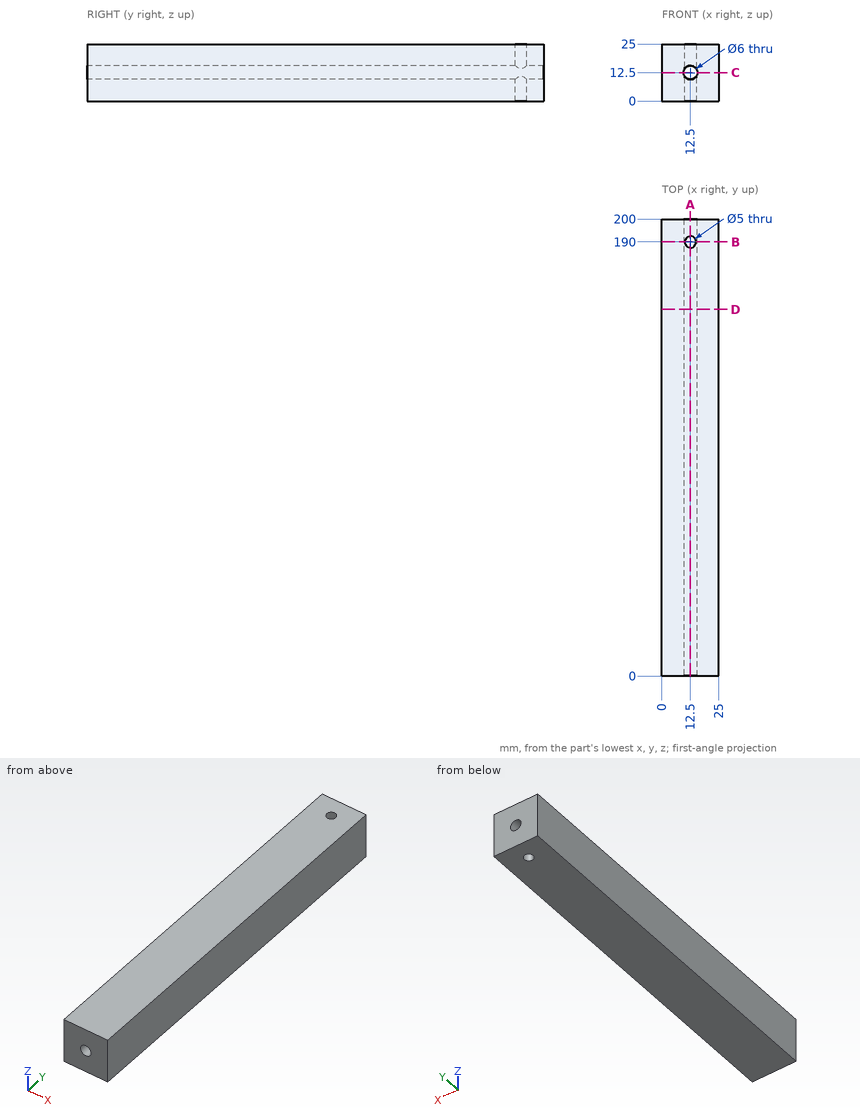
Part print with two shaded views. Sizes in mm from the minimum x, y, z corner. Coordinates: 2 decimals unless noted, no trailing zeros. Write each loop counter-clockwise with the first axis right and the second up, starting at its lowest first coordinate (ties: lowest second). Pieces come first, ordered by that corner, then holes. Notation, with made-up numbers: (15.25, 89.5) - (67.25, 89.5) arc R9 cw to (67.25, 100.5) - close; hole circle Ø2 at (42.5, 9). An arc over 180 degrees is marked (long way). Put each result on its own line as item: value.
1. Band-saw the part on B-B (y = 190). Write the cut outline in (x, z), then the cut area to 3 significant figures.
Final values:
outline: (0, 0) - (10, 0) - (10, 10.84) arc R3 cw to (10, 14.16) - (10, 25) - (0, 25) - close; (15, 0) - (25, 0) - (25, 25) - (15, 25) - (15, 14.16) arc R3 cw to (15, 10.84) - close
area: 498 mm²
2. Flat gauge pin, fed straight in: pin 1 Ø4.5 at (x, y) = (12.5, 190) entering from -Z. Where does the tip first touch, or does it go through?
Final values:
pin 1: passes through
3. Band-saw the part on A-A (x = 12.5). Write the cut outline in (y, z).
Final values:
outline: (0, 0) - (187.5, 0) - (187.5, 9.5) - (0, 9.5) - close; (0, 15.5) - (187.5, 15.5) - (187.5, 25) - (0, 25) - close; (192.5, 0) - (200, 0) - (200, 9.5) - (192.5, 9.5) - close; (192.5, 15.5) - (200, 15.5) - (200, 25) - (192.5, 25) - close
4. Band-saw the part on C-C (z = 12.5). Write the cut outline in (x, y), then the cut area to 3 significant figures.
Final values:
outline: (0, 0) - (9.5, 0) - (9.5, 200) - (0, 200) - close; (15.5, 0) - (25, 0) - (25, 200) - (15.5, 200) - close
area: 3,800 mm²
5. Probe line 1 along Z through (x, y) = (12.5, 80.5); line 2 along Y through (x, z) = (12.5, 16.5); line 3 along X through (y, z) = (36, 10). List the from-to ranges inside material, lowest first. Write a range as [from, to].
Final values:
line 1: z = [0, 9.5], [15.5, 25]
line 2: y = [0, 187.5], [192.5, 200]
line 3: x = [0, 10.84], [14.16, 25]
6. Band-saw the part on D-D (y = 160.5). Write the cut outline in (x, z), then the cut area to 3 significant figures.
Final values:
outline: (0, 0) - (25, 0) - (25, 25) - (0, 25) - close; hole circle Ø6 at (12.5, 12.5)
area: 597 mm²
